Part model, mm, in its own coordinate system. A direction names the side the tool comes from. Coordinates: 2 decimals unless noted, no trailing zeros. Loops run counter-clockwise (first coordinate to the right, second up) from the corner with the lowest first, then second, coordinate; pieces in that order, holes last. Notation, with made-up numbers: M 70,-19 L 117,-19 A11 cw 117,-3 Z; hole C -15,-23 d4. An arc over 180 degrees is marked long. Answer as a JSON object with one key per item and string values. Group by question number.
1. Saw through at D-D on z = -13.5. Write the cut outline in (x, y).
2. Saw through at A-A on x = 29. Write the cut outline in (y, z), then the cut area to 3 significant figures.
3. Drop a flat-ended pin along its axis: pin 1 Ø17.5 at (x, z) = (-4, 8.5) entering from +Y. Give the stop position or say it passes through.
4. 3-axis set-ups, long thin cutter, end or side, ignore diameter. For faces 4 (the face through (-7, 13, 17.5)), 5 (the face through (-40, 11, 0)), 6 (the face through (36, 9, -2)): which of +Z, -Z, +X, -X, +Y, -Y reach the whole face in a straight line?
5. Saw through at C-C on y = 7.5. Write the cut outline in (x, z).
6. Drill centre lines: L1, parallel to X at y = 14.75, z = -7.5; L2, parallel to Z at x = 12, y = 21.25; L3, parallel to X at y = 1.25, z = -6. Where is each one in solid material? Low to high.
7. Saw through at B-B on z = 16.5. Write the cut outline in (x, y).
8. Mould opens along Z. For faces 1 (the face through (0, 1, -12)), 2 (the face through (-1, 0, -15)), 3 (the face through (-1, 11, 22)) say: released by +Z, released by -Z, zero draft, split by the parting line, or undercut.
from build123d import *

# Parameters (mm, degrees)
SKETCH1_W           = 80
SKETCH1_H           = 44
SKETCH1_W_2         = 60
SKETCH1_H_2         = 24
BOSS_EXTRUDE1_DEPTH = 3
SKETCH2_W           = 80
SKETCH2_H           = 44
SKETCH2_W_2         = 71
SKETCH2_H_2         = 35
BOSS_EXTRUDE2_DEPTH = 20
CUT_EXTRUDE1_REACH  = 53.118
SKETCH3_W           = 15
SKETCH3_H           = 20


with BuildPart() as part:
    # Sketch1 → Boss-Extrude1 (new body)
    with BuildSketch(Plane(origin=(0, 0, 0), x_dir=(1, 0, 0), z_dir=(0, 1, 0))):
        Rectangle(SKETCH1_W, SKETCH1_H)
        Rectangle(SKETCH1_W_2, SKETCH1_H_2, mode=Mode.SUBTRACT)
    extrude(amount=BOSS_EXTRUDE1_DEPTH)

    # Sketch2 → Boss-Extrude2 (add)
    with BuildSketch(Plane(origin=(0, 3, 0), x_dir=(1, 0, 0), z_dir=(0, 1, 0))):
        Rectangle(SKETCH2_W, SKETCH2_H)
        Rectangle(SKETCH2_W_2, SKETCH2_H_2, mode=Mode.SUBTRACT)
    extrude(amount=BOSS_EXTRUDE2_DEPTH)

    # Sketch3 → Cut-Extrude1 (cut, up to next)
    with BuildSketch(Plane(origin=(0, 0, 0), x_dir=(-1, 0, 0), z_dir=(0, -1, 0)), mode=Mode.PRIVATE) as cut_extrude1_sk1:
        with Locations((-30.5, -8)):
            Rectangle(SKETCH3_W, SKETCH3_H)
    cut_extrude1_tool1 = extrude(cut_extrude1_sk1.sketch, amount=-CUT_EXTRUDE1_REACH, mode=Mode.PRIVATE) & part.part
    add(cut_extrude1_tool1.solids().sort_by_distance((30.5, 0, 8))[0], mode=Mode.SUBTRACT)


solid = part.part
Outcome:
{
 "1": {"outline": "M -40,0 L 40,0 L 40,23 L 35.5,23 L 35.5,3 L -35.5,3 L -35.5,23 L -40,23 Z"},
 "2": {"outline": "M 0,-22 L 23,-22 L 23,-17.5 L 3,-17.5 L 3,-12 L 0,-12 Z; M 0,18 L 23,18 L 23,22 L 0,22 Z", "area": "212 mm²"},
 "3": {"pin 1": "stops at y = 3"},
 "4": {"face 4": "+Y", "face 5": "+Z, -Z, -X, +Y, -Y", "face 6": "+Y, -Y"},
 "5": {"outline": "M -40,-22 L 40,-22 L 40,22 L -40,22 Z; hole M -35.5,-17.5 L 35.5,-17.5 L 35.5,-2 L 38,-2 L 38,18 L 23,18 L 23,17.5 L -35.5,17.5 Z"},
 "6": {"L1": "x = -40 to -35.5, 35.5 to 40", "L2": "z = -22 to -17.5, 17.5 to 22", "L3": "x = -40 to -30, 30 to 40"},
 "7": {"outline": "M -40,0 L 23,0 L 23,3 L -35.5,3 L -35.5,23 L -40,23 Z; M 38,0 L 40,0 L 40,23 L 38,23 Z"},
 "8": {"face 1": "undercut", "face 2": "zero draft", "face 3": "released by +Z"}
}
